Geometry: final body of the model. Coordinates: model frame, mm. A direction names the side the tool comes from. Coordinates: 2 decimals unless noted, no trailing zeros. Loops run counter-clockwise (first coordinate to the right, second up) from the corner with the lowest first, then second, coordinate; pieces in that order, holes last. Notation, with made-up numbers: (69, -18.5) - (90, -18.5) arc R20 ccw to (90, -6.5) - close; hole circle Ø9 at (61, 46.5). An arc over 180 degrees is marked (long way). Return JSON: item names as keys, results as strings.
from build123d import *

# Parameters (mm, degrees)
F0_W     = 2
F0_H     = 2
F1_DEPTH = 8
F2_ANGLE = 180
F0_W_2   = 1.5
F0_W_3   = 3
F3_DEPTH = 2


with BuildPart() as f1:
    # F0 (on Front) → F1 (new body, symmetric)
    with BuildSketch(Plane.XZ):
        with Locations((3.5, 7.2)):
            Rectangle(F0_W, F0_H)
        Polygon((4.5, 1.2), (6, 1.2), (6, 8.2), (4.5, 8.2), (4.5, 6.2), align=None)
        Polygon((-6, -1.2), (6, -1.2), (6, 1.2), (4.5, 1.2), (-6, 1.2), align=None)
    extrude(amount=F1_DEPTH, both=True)

    # F0 (on Front) → F2 (revolve, symmetric)
    with BuildSketch(Plane.XZ) as f2_sk:
        Polygon((-14, -1.2), (-6, -1.2), (-6, 1.2), (-11, 1.2), (-14, 1.2), align=None)
    revolve(axis=Axis((-6, 0, 0), (0, 0, 1)), revolution_arc=F2_ANGLE / 2)
    revolve(f2_sk.sketch, axis=Axis((-6, 0, 0), (0, 0, -1)), revolution_arc=F2_ANGLE / 2)

    # F0 (on Front) → F3 (join, symmetric)
    with BuildSketch(Plane.XZ):
        with Locations((-14.75, 2.2)):
            Rectangle(F0_W_2, F0_H)
        with Locations((-12.5, 2.2)):
            Rectangle(F0_W_3, F0_H)
    extrude(amount=F3_DEPTH, both=True)


solid = f1.part
Item 1: First-contact query: pin 1 Ø1.6 at (x, z) = (-13.5, 2.5) entering from -Y; pin 2 Ø1.4 at (x, y) = (-15, 0) entering from -Z; pin 3 Ø4.5 at (x, y) = (-12.5, -0.5) entering from +Z. Flat tips, straight axial feed; report the tip coordinate or a pass-through.
Worked out:
{"pin 1": "y = -2", "pin 2": "z = 1.2", "pin 3": "z = 3.2"}
Item 2: Section query C-C, the plane y = 0. Return loops of the section in (x, z).
Worked out:
{"outline": "(-15.5, 1.2) - (-14, 1.2) - (-14, -1.2) - (6, -1.2) - (6, 8.2) - (2.5, 8.2) - (2.5, 6.2) - (4.5, 6.2) - (4.5, 1.2) - (-11, 1.2) - (-11, 3.2) - (-15.5, 3.2) - close"}
Item 3: Ray query, probe 1 along X at (y, z) = (-0.75, 2.25); probe 2 along Z at (x, y) = (3, -7); probe 3 along Z at (x, y) = (-5, 4). Return the intervals inside material, ascending. Write a range as from..to.
Worked out:
{"probe 1": "-15.5..-11, 4.5..6", "probe 2": "-1.2..1.2, 6.2..8.2", "probe 3": "-1.2..1.2"}
Item 4: Reachability of faces 4 (the face through (-13, -2, 2)), 5 (the face through (4.5, 0, 4)), 6 (the face through (-13, 0, 3.2)) from +Z, -Z, +X, -X, +Y, -Y: full face, straight path, thin tool, end or side. Return the list, or none.
Worked out:
{"face 4": "+Z, -X, -Y", "face 5": "+Y, -Y", "face 6": "+Z, -X, +Y, -Y"}
Item 5: Mould query, pull axis X, two halves, no side actions, for faces 1 (the face through (-14, 0, 0)), 2 (the face through (3, 0, 6.2)), 3 (the face through (-11, 0, 2)). Classes: +X half, -X half, draft (parallel to the pull), parting line (faces both ways), or undercut.
Worked out:
{"face 1": "-X half", "face 2": "draft", "face 3": "undercut"}
Item 6: Section query B-B, the plane x = 4.25. Return loops of the section in (y, z), and give its area (3 significant figures).
Worked out:
{"outline": "(-8, -1.2) - (8, -1.2) - (8, 1.2) - (-8, 1.2) - close; (-8, 6.2) - (8, 6.2) - (8, 8.2) - (-8, 8.2) - close", "area": "70.4 mm^2"}
Item 7: Section query A-A, the plane z = 2. Return loops of the section in (x, y), and give its area (3 significant figures).
Worked out:
{"outline": "(-15.5, -2) - (-11, -2) - (-11, 2) - (-15.5, 2) - close; (4.5, -8) - (6, -8) - (6, 8) - (4.5, 8) - close", "area": "42.0 mm^2"}
Item 8: Section query D-D, the plane x = -12.25. Return loops of the section in (y, z).
Worked out:
{"outline": "(-4.99, -1.2) - (4.99, -1.2) - (4.99, 1.2) - (2, 1.2) - (2, 3.2) - (-2, 3.2) - (-2, 1.2) - (-4.99, 1.2) - close"}
